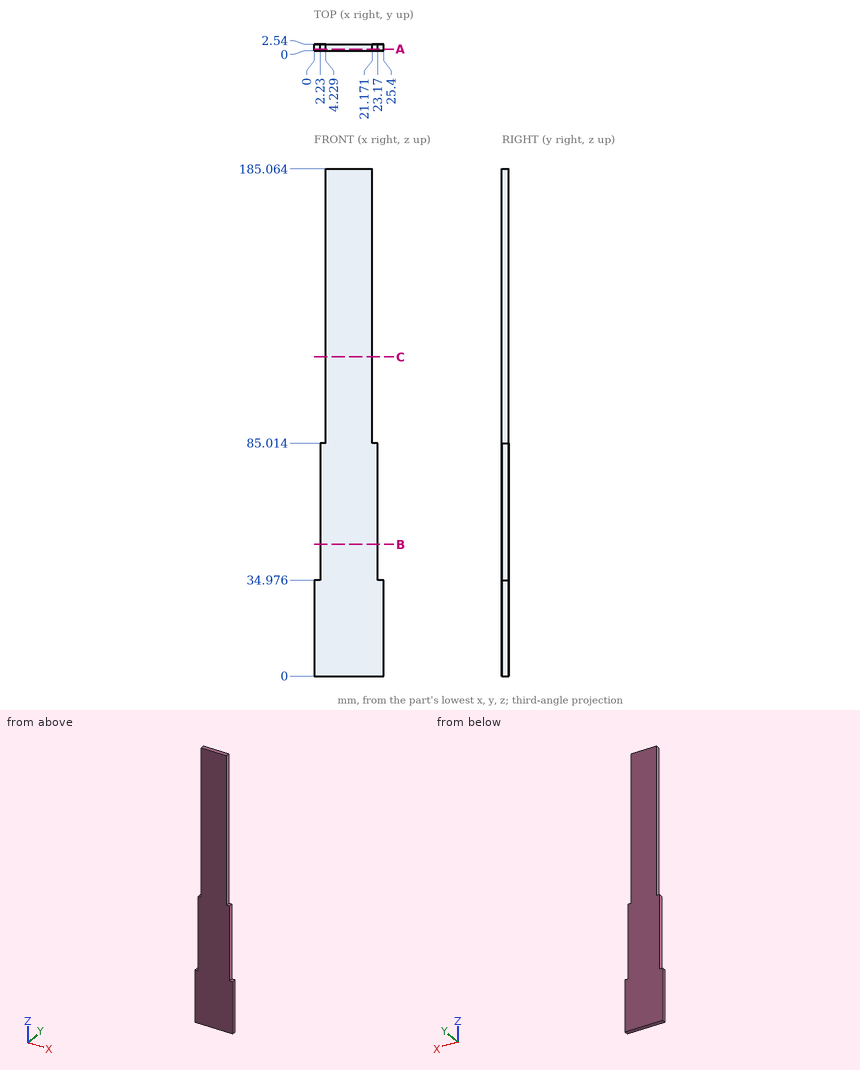
Source: three-view drawing plus pictorial views. Frame: mm from the lowest corner of the part. Round coordinates to 2 decimals unless told otherwise and drop trailing zeros. Loops run counter-clockwise (first coordinate to the right, second up) from the corner with the lowest first, then second, coordinate; pieces in that order, holes last. Notation, with made-up numbers: (-8.75, 6) -> (22.25, 6) arc R11 cw to (22.25, 11) -> close; hole circle Ø6 at (45.25, -27.5). An arc over 180 degrees is marked (long way). Use one line per item in the form item = value.
Item 1: Cut plane B-B on z = 48. Output: boundary loops of the cut face in (x, y).
Evaluation:
outline = (2.23, 0) -> (23.17, 0) -> (23.17, 2.54) -> (2.23, 2.54) -> close
Item 2: Contact query for flat-ended pins moving along their axis: pin 1 Ø5 at (x, z) = (3.5, 37.5) entering from -Y; pin 2 Ø1 at (x, y) = (22, 2) entering from +Z; pin 3 Ø0.8 at (y, z) = (1.5, 151) entering from +X; pin 4 Ø1.1 at (x, y) = (24, 1.5) entering from +Z. Output: stop coordinate, or through.
Evaluation:
pin_1 = 0
pin_2 = 85.01
pin_3 = 21.17
pin_4 = 34.98
Item 3: Cut plane C-C on z = 116.5. Output: boundary loops of the cut face in (x, y).
Evaluation:
outline = (4.23, 0) -> (21.17, 0) -> (21.17, 2.54) -> (4.23, 2.54) -> close
Item 4: Material intervals for probe 1 along X at (y, z) = (2.4, 55); probe 2 along Z at (x, y) = (22.25, 0.6); probe 3 along X at (y, z) = (0.35, 124.5), sorted ascending.
Evaluation:
probe_1 = 2.23 to 23.17
probe_2 = 0 to 85.01
probe_3 = 4.23 to 21.17
Item 5: Cut plane A-A on y = 0.65. Output: boundary loops of the cut face in (x, z) (1 decimal), then the cut area to 3 significant figures.
Evaluation:
outline = (0, 0) -> (25.4, 0) -> (25.4, 35) -> (23.2, 35) -> (23.2, 85) -> (21.2, 85) -> (21.2, 185.1) -> (4.2, 185.1) -> (4.2, 85) -> (2.2, 85) -> (2.2, 35) -> (0, 35) -> close
area = 3,630 mm2
